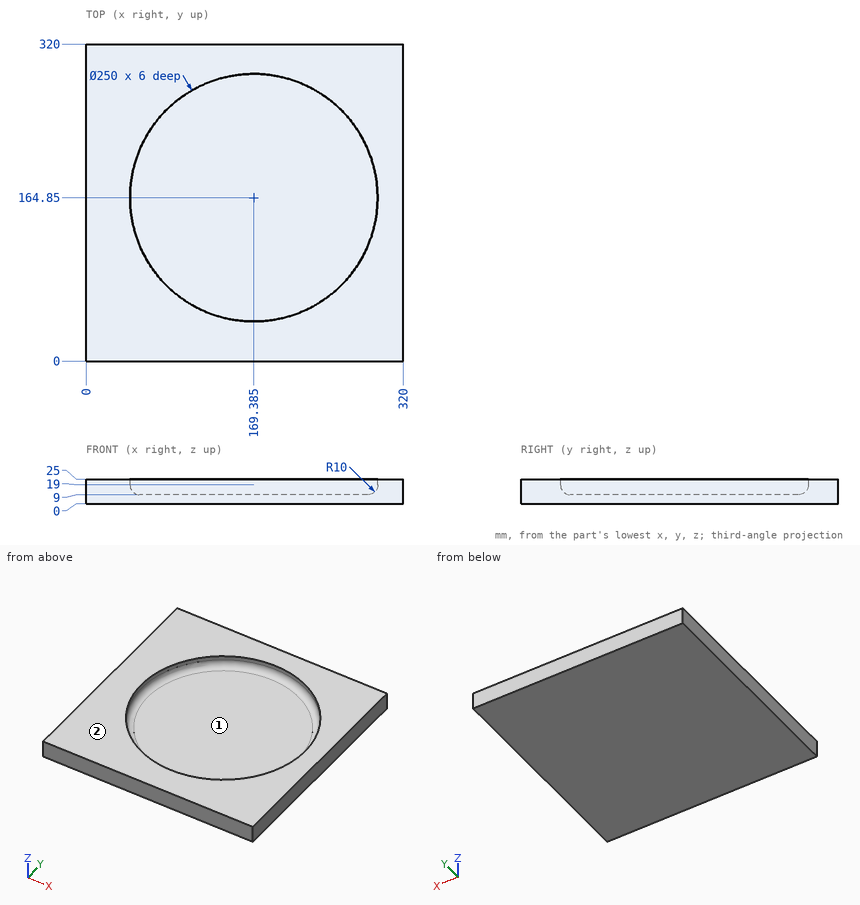
Geometry check sheet. Reference: drawing and pictorial views, mm from the part's lowest x, y, z. Round coordinates to 2 decimals unless told otherwise and drop trailing zeros. Write item = value, one per line.
Q1. Scan lines: line 1 (Y direction, x = 85.5, z = 14) (1 decimal); line 2 (Z direction, x = 82, y = 229.5); line 3 (Y direction, x = 269.5, z = 16.25). Record each from-to range of solid material in increasing order.
Answer block:
line_1 = 0 to 74, 255.7 to 320
line_2 = 0 to 9
line_3 = 0 to 90.65, 239.05 to 320
Q2. Release check for a two-part mould opening along Y. For the marked faces 1 and 2 record: released by +Y, released by -Y, zero draft, split by the parting line, or undercut.
Answer block:
face_1 = undercut
face_2 = zero draft
Q3. Depth check by flat-ended pin: pin 1 Ø6 at (x, y) = (145.5, 53.5) entering from +Z; pin 2 Ø5 at (x, y) = (232, 205.5) entering from +Z. Enter the tip coordinate at first touch or a pass-through.
Answer block:
pin_1 = 9.18
pin_2 = 9
